from build123d import *

# Parameters (mm, degrees)
SKETCH2_W           = 46
SKETCH2_H           = 32
SKETCH2_R           = 1.525
SKETCH2_R_2         = 7
BOSS_EXTRUDE1_DEPTH = 5
SKETCH3_R           = 3.8
CUT_EXTRUDE1_DEPTH  = 2.5
BOSS_EXTRUDE2_DEPTH = 87.8
BOSS_EXTRUDE3_START = 82.8
SKETCH2_2_W         = 46
SKETCH2_2_H         = 32
SKETCH2_2_R         = 1.525
SKETCH2_2_R_2       = 7
BOSS_EXTRUDE3_DEPTH = 5
CUT_EXTRUDE2_START  = 80.3
SKETCH3_3_R         = 3.8
CUT_EXTRUDE2_DEPTH  = 2.5
CUT_EXTRUDE3_DEPTH  = 5
CUT_EXTRUDE4_DEPTH  = 5


with BuildPart() as part:
    # Sketch2 → Boss-Extrude1 (new body)
    with BuildSketch(Plane(origin=(0, 0, 0), x_dir=(1, 0, 0), z_dir=(0, 1, 0))):
        Rectangle(SKETCH2_W, SKETCH2_H)
        with Locations(Location((-17, 9, 0), (0, 0, 270))):
            Circle(SKETCH2_R, mode=Mode.SUBTRACT)
        with Locations(Location((-17, -9, 0), (0, 0, 270))):
            Circle(SKETCH2_R, mode=Mode.SUBTRACT)
        with Locations(Location((16, -9, 0), (0, 0, 270))):
            Circle(SKETCH2_R, mode=Mode.SUBTRACT)
        with Locations(Location((16, 9, 0), (0, 0, 270))):
            Circle(SKETCH2_R, mode=Mode.SUBTRACT)
        with Locations(Location((-8, 0, 0), (0, 0, 270))):
            Circle(SKETCH2_R_2, mode=Mode.SUBTRACT)
    extrude(amount=BOSS_EXTRUDE1_DEPTH)

    # Sketch3 → Cut-Extrude1 (cut)
    with BuildSketch(Plane(origin=(0, 5, 0), x_dir=(1, 0, 0), z_dir=(0, 1, 0))):
        with Locations(Location((-17, 9, 0), (0, 0, 270))):
            Circle(SKETCH3_R)
        with Locations(Location((-17, -9, 0), (0, 0, 270))):
            Circle(SKETCH3_R)
        with Locations(Location((16, -9, 0), (0, 0, 270))):
            Circle(SKETCH3_R)
        with Locations(Location((16, 9, 0), (0, 0, 270))):
            Circle(SKETCH3_R)
        with BuildLine():
            Line((7.5, 5), (7.5, -5))
            ThreePointArc((7.5, -5), (5, -7.5), (2.5, -5))
            Line((2.5, -5), (2.5, 5))
            ThreePointArc((2.5, 5), (5, 7.5), (7.5, 5))
        make_face()
    extrude(amount=-CUT_EXTRUDE1_DEPTH, mode=Mode.SUBTRACT)

    # Sketch4 → Boss-Extrude2 (add)
    with BuildSketch(Plane(origin=(0, 0, 0), x_dir=(-1, 0, 0), z_dir=(0, -1, 0))):
        Polygon((23, 16), (-23, 16), (-23, -16), (-27, -16), (-27, 18.5), (27, 18.5), (27, -16), (23, -16), align=None)
    extrude(amount=-BOSS_EXTRUDE2_DEPTH)

    # Sketch2<2> → Boss-Extrude3 (add)
    with BuildSketch(Plane(origin=(0, 0, 0), x_dir=(1, 0, 0), z_dir=(0, 1, 0)).offset(BOSS_EXTRUDE3_START)):
        Rectangle(SKETCH2_2_W, SKETCH2_2_H)
        with Locations(Location((-17, 9, 0), (0, 0, 270))):
            Circle(SKETCH2_2_R, mode=Mode.SUBTRACT)
        with Locations(Location((-17, -9, 0), (0, 0, 270))):
            Circle(SKETCH2_2_R, mode=Mode.SUBTRACT)
        with Locations(Location((16, -9, 0), (0, 0, 270))):
            Circle(SKETCH2_2_R, mode=Mode.SUBTRACT)
        with Locations(Location((16, 9, 0), (0, 0, 270))):
            Circle(SKETCH2_2_R, mode=Mode.SUBTRACT)
        with Locations(Location((-8, 0, 0), (0, 0, 270))):
            Circle(SKETCH2_2_R_2, mode=Mode.SUBTRACT)
    extrude(amount=BOSS_EXTRUDE3_DEPTH)

    # Sketch3<3> → Cut-Extrude2 (cut)
    with BuildSketch(Plane(origin=(0, 5, 0), x_dir=(1, 0, 0), z_dir=(0, 1, 0)).offset(CUT_EXTRUDE2_START)):
        with Locations(Location((-17, 9, 0), (0, 0, 270))):
            Circle(SKETCH3_3_R)
        with Locations(Location((-17, -9, 0), (0, 0, 270))):
            Circle(SKETCH3_3_R)
        with Locations(Location((16, -9, 0), (0, 0, 270))):
            Circle(SKETCH3_3_R)
        with Locations(Location((16, 9, 0), (0, 0, 270))):
            Circle(SKETCH3_3_R)
        with BuildLine():
            Line((7.5, 5), (7.5, -5))
            ThreePointArc((7.5, -5), (5, -7.5), (2.5, -5))
            Line((2.5, -5), (2.5, 5))
            ThreePointArc((2.5, 5), (5, 7.5), (7.5, 5))
        make_face()
    extrude(amount=-CUT_EXTRUDE2_DEPTH, mode=Mode.SUBTRACT)

    # Sketch5 → Cut-Extrude3 (cut)
    with BuildSketch(Plane(origin=(27, 0, 0), x_dir=(0, 0, -1), z_dir=(1, 0, 0))):
        Polygon((-16, 43.9), (-16, 5), (4, 5), (16, 17.9), (16, 43.9), align=None)
        Polygon((-16, 82.8), (-16, 43.9), (16, 43.9), (16, 73.9), (7, 82.8), align=None)
    extrude(amount=-CUT_EXTRUDE3_DEPTH, mode=Mode.SUBTRACT)

    # Sketch6 → Cut-Extrude4 (cut)
    with BuildSketch(Plane.ZY.offset(27)):
        Polygon((16, 82.8), (16, 5), (-16, 29), (-16, 58.8), align=None)
    extrude(amount=-CUT_EXTRUDE4_DEPTH, mode=Mode.SUBTRACT)


solid = part.part
Could you check a few things on this model? Use its own coordinates, in mm. A direction names the side the tool comes from. Give positions to 0.01 mm unless a question says otherwise; leave off trailing zeros. Order: outer loops, then holes, each group sorted by start corner. A loop starts at its lowest first (then second) coordinate and runs counter-clockwise, first axis right, second up. Notation, with made-up numbers: (18, -33.75) -> (73, -33.75) arc R32 ccw to (73, -4.75) -> close; hole circle Ø3 at (16.5, 62). An arc over 180 degrees is marked (long way). Return JSON: item names as keys, results as strings.
1. Imagine slicing it at D-D on y = 20. List the corners of the cut face in (x, z) for me.
Answer list:
{"outline": "(-27, -18.5) -> (27, -18.5) -> (27, -16) -> (-23, -16) -> (-23, -4) -> (-27, -4) -> close"}
2. On a 3-axis mill with a long thin cutter (end or side, diameter ignored), from which of +Z, -Z, +X, -X, +Y, -Y can I reach the whole of each face in a straight line? I mean faces 5 (the cylindrical face through (-18.49, 86.53, 8.67)), 6 (the flat face through (5, 2.5, 0)), 7 (the flat face through (-25, 17, 0)). Say none if no direction works.
Answer list:
{"face 5": "+Y, -Y", "face 6": "none", "face 7": "+Z, +X, -X"}
3. I need wall thicknesses on line 1 (Z direction, x = -17, y = 85.85) (3 decimals); line 2 (X direction, y = 86.4, z = 9) (3 decimals); line 3 (X direction, y = 3, z = -9). Which ranges of each line are inside material? Lowest first, please. Write a range as from..to.
Answer list:
{"line 1": "z = -18.5..-10.525, -7.475..7.475, 10.525..16", "line 2": "x = -27..-18.525, -15.475..14.475, 17.525..27", "line 3": "x = -27..-20.8, -13.2..12.2, 19.8..27"}
4. Imagine slicing it at B-B on x = -8. List the corners of the cut face in (y, z) for me.
Answer list:
{"outline": "(0, -18.5) -> (87.8, -18.5) -> (87.8, -7) -> (82.8, -7) -> (82.8, -16) -> (5, -16) -> (5, -7) -> (0, -7) -> close; (0, 7) -> (5, 7) -> (5, 16) -> (0, 16) -> close; (82.8, 7) -> (87.8, 7) -> (87.8, 16) -> (82.8, 16) -> close"}
5. Imagine slicing it at C-C on x = 11. List the corners of the cut face in (y, z) for me.
Answer list:
{"outline": "(0, -18.5) -> (87.8, -18.5) -> (87.8, 16) -> (82.8, 16) -> (82.8, -16) -> (5, -16) -> (5, 16) -> (0, 16) -> close"}
6. Imagine slicing it at A-A on z = 0. List the corners of the cut face in (x, y) for me, then the cut area to 3 significant figures.
Answer list:
{"outline": "(-27, 0) -> (-15, 0) -> (-15, 5) -> (-23, 5) -> (-23, 17) -> (-27, 17) -> close; (-27, 70.8) -> (-23, 70.8) -> (-23, 82.8) -> (-15, 82.8) -> (-15, 87.8) -> (-27, 87.8) -> close; (-1, 0) -> (27, 0) -> (27, 5) -> (7.5, 5) -> (7.5, 2.5) -> (2.5, 2.5) -> (2.5, 5) -> (-1, 5) -> close; (-1, 82.8) -> (2.5, 82.8) -> (2.5, 85.3) -> (7.5, 85.3) -> (7.5, 82.8) -> (27, 82.8) -> (27, 87.8) -> (-1, 87.8) -> close", "area": "471 mm2"}
7. For pin 1 Ø4.5 at (x, z) = (-17, -9) entering from +Y, with a flat end and sliding along its axis, tell me the tip position at first contact or that it passes through.
Answer list:
{"pin 1": "stops at y = 87.8"}
8. Thinking about a two-plate mould opening in X: for faces 1 (the flat face through (0, 2, 16)), 2 (the cylindrical face through (-14.834, 85.265, -1.517)), 3 (the cylindrical face through (-19.312, 84.068, 5.984)), 4 (the flat face through (27, 34, -17)), which applies, pulls with the +X half, pulls with the -X half, needs draft (parallel to the pull), parting line crosses it, or undercut?
Answer list:
{"face 1": "needs draft", "face 2": "undercut", "face 3": "undercut", "face 4": "pulls with the +X half"}
